Part print with two shaded views. Sizes in mm from the minimum x, y, z corner. A direction names the side the tool comes from. Give positions to 0.01 mm unless a question says otherwise; leave off trailing zeros. Loops run counter-clockwise (first coordinate to the right, second up) from the corner with the lowest first, then second, coordinate; pieces in that order, holes last. Notation, with made-up numbers: M 25,10 L 80,10 A15 ccw 80,38 Z; hole C -40,-9 d9. An arc over 180 degrees is marked long. Answer in a Markdown table with one row per item.
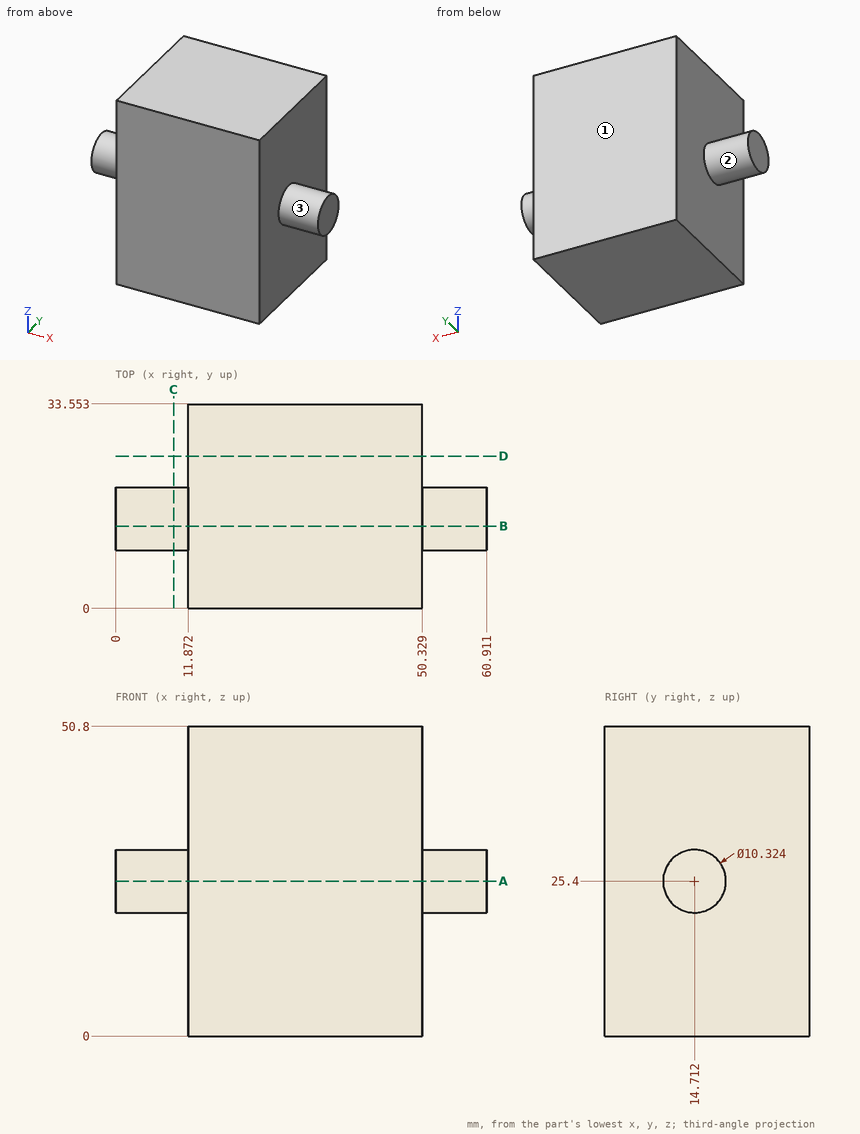
Q1. Probe probe 1 along X at (y, z) = (8, 20); probe 2 along Z at (x, y) = (50.5, 12); probe 3 along Z at (x, y) = (58.5, 17) (1 decimal). List the from-to ranges inside material, lowest first.
Reported:
| item | result |
|---|---|
| probe 1 | 11.87 to 50.33 |
| probe 2 | 21.01 to 29.79 |
| probe 3 | 20.8 to 30 |
Q2. 3-axis set-ups, long thin cutter, end or side, ignore diameter. For the marked faces 1, 2 and 3: which of +Z, -Z, +X, -X, +Y, -Y reach the whole face in a straight line?
Reported:
| item | result |
|---|---|
| face 1 | +Z, -Z, +X, -X, +Y |
| face 2 | -X |
| face 3 | +X |
Q3. Saw through at D-D (y = 25). Give the cut face in (x, z).
Reported:
| item | result |
|---|---|
| outline | M 11.87,0 L 50.33,0 L 50.33,50.8 L 11.87,50.8 Z |
Q4. Saw through at B-B (y = 13.5). Give the cut face in (x, z), and give its area (3 significant figures).
Reported:
| item | result |
|---|---|
| outline | M 0,20.38 L 11.87,20.38 L 11.87,0 L 50.33,0 L 50.33,20.38 L 60.91,20.38 L 60.91,30.42 L 50.33,30.42 L 50.33,50.8 L 11.87,50.8 L 11.87,30.42 L 0,30.42 Z |
| area | 2,180 mm² |
Q5. Saw through at C-C (x = 9.5). Give the cut face in (y, z), and give its area (3 significant figures).
Reported:
| item | result |
|---|---|
| outline | C 14.71,25.4 d10.32 |
| area | 83.7 mm² |
Q6. Drop flat-ended pins along their axis: pin 1 (10 mm diameter, centred on x = 24.5, y = 15.5, fed in from -Z); pin 2 (1 mm diameter, centred on x = 11, z = 17, fed in from -Y); pin 3 (3 mm diameter, centred on y = 21.5, z = 41, fed in from +X); pin 4 (1 mm diameter, centred on y = 12, z = 15, fed in from -X). Give the stop position or say it passes through.
Reported:
| item | result |
|---|---|
| pin 1 | z = 0 |
| pin 2 | through |
| pin 3 | x = 50.33 |
| pin 4 | x = 11.87 |
Q7. Saw through at A-A (z = 25.4). Give the cut face in (x, y), and give its area (3 significant figures).
Reported:
| item | result |
|---|---|
| outline | M 0,9.55 L 11.87,9.55 L 11.87,0 L 50.33,0 L 50.33,9.55 L 60.91,9.55 L 60.91,19.87 L 50.33,19.87 L 50.33,33.55 L 11.87,33.55 L 11.87,19.87 L 0,19.87 Z |
| area | 1,520 mm² |
